Geometry: final body of the model. Coordinates: model frame, mm. Face numbers are marked on the shaded views. Give positions to 0.01 mm unless a question says otherwise; leave off trailing zeros. Write each loop counter-clockwise with the first axis right and the second up, starting at its lowest first coordinate (ties: lowest second). Pieces come first, ordered by that corner, then holes. Notation, with made-up numbers: M 38.25,52 L 49.25,52 A24 cw 49.25,84 Z; hole C 25.25,49 d7. An arc over 180 degrees is marked long. Use a Markdown table: item, result. Add a question column.
1) Section A-A on y = -37. Return the cut outline in (x, z), then the cut area to 3 significant figures.
2) Draft query along X for the marked faces 1, 2, 3 and 4. Return one class per face: +X half, -X half, draft (parallel to the pull), parting line (faces both ways), or undercut.
3) Section D-D on x = 15.5. Return the cut outline in (y, z).
4) Pin query (flat end, axial travel): pin 1 (7 mm diameter, centred on y = -28, z = 61, fed in from -X); pin 2 (1 mm diameter, centred on y = -32.5, z = 47, fed in from +X); pin 3 (12 mm diameter, centred on x = 28, y = -5, fed in from -Z); pin 4 (3 mm diameter, centred on x = 15, y = -7, fed in from -Z). Return the tip coordinate at first contact, or that it passes through.
5) Section C-C on x = -26. Return the cut outline in (y, z), then the cut area to 3 significant figures.
6) Section B-B on z = 59.75. Return the cut outline in (x, y).
7) Line query: line 1 (Y direction, x = 0, z = 55.75); line 2 (X direction, y = -15, z = 50.75); line 3 (X direction, y = -42.5, z = 44). Output: solid intervals per line, ascending.
```python
from build123d import *

# Parameters (mm, degrees)
F3_DEPTH  = 50
F7_DEPTH  = 10
F9_D      = 4.2
F9_DEPTH  = 4.8
F9_TIP    = 1.2618073
F11_D     = 7
F11_DEPTH = 28
F11_TIP   = 2.1030121666


with BuildPart() as f3:
    # F2 (on Front) → F3 (new body)
    with BuildSketch(Plane.XZ):
        with BuildLine():
            ThreePointArc((-26.8236083475, 42.1046311493), (-13.9699038675, 47.9285688805), (0, 49.923))
            Line((0, 49.923), (0, 59))
            Line((0, 59), (-7.5, 59))
            Line((-7.5, 59), (-7.5, 65.5724789832))
            ThreePointArc((-7.5, 65.5724789832), (-22.044813763, 62.2095345277), (-35.4617741509, 55.6638354237))
            Line((-35.4617741509, 55.6638354237), (-26.8236083475, 42.1046311493))
        make_face()
        with BuildLine():
            ThreePointArc((0, 49.923), (13.9699038675, 47.9285688805), (26.8236083475, 42.1046311493))
            Line((26.8236083475, 42.1046311493), (35.4617741509, 55.6638354237))
            ThreePointArc((35.4617741509, 55.6638354237), (22.044813763, 62.2095345277), (7.5, 65.5724789832))
            Line((7.5, 65.5724789832), (7.5, 59))
            Line((7.5, 59), (0, 59))
            Line((0, 59), (0, 49.923))
        make_face()
    extrude(amount=F3_DEPTH)

    # F6 (on line) → F7 (cut)
    with BuildSketch(Plane(origin=(20.9552129656, 0, 45.1351855936), x_dir=(0.9070121064, 0, -0.4211045463), z_dir=(0.4211045463, 0, 0.9070121064))):
        with BuildLine():
            ThreePointArc((3, -47.5), (3.7071067812, -47.2071067812), (4, -46.5))
            Line((4, -46.5), (4, -3.5))
            ThreePointArc((4, -3.5), (3.7071067812, -2.7928932188), (3, -2.5))
            Line((3, -2.5), (-3, -2.5))
            ThreePointArc((-3, -2.5), (-3.7071067812, -2.7928932188), (-4, -3.5))
            Line((-4, -3.5), (-4, -46.5))
            ThreePointArc((-4, -46.5), (-3.7071067812, -47.2071067812), (-3, -47.5))
            Line((-3, -47.5), (3, -47.5))
        make_face()
    extrude(amount=F7_DEPTH, mode=Mode.SUBTRACT)

    # F9
    with Locations(Plane.XY.offset(59)):
        with Locations((0, -25)):
            Hole(F9_D / 2, depth=F9_DEPTH)
            with Locations((0, 0, -(F9_DEPTH + F9_TIP / 2))):  # 118° drill point
                Cone(0, F9_D / 2, F9_TIP, mode=Mode.SUBTRACT)

    # F11
    with Locations(Plane.XZ.offset(50)):
        with Locations((23.4093313461, 50.6118115303)):
            Hole(F11_D / 2, depth=F11_DEPTH)
            with Locations((0, 0, -(F11_DEPTH + F11_TIP / 2))):  # 118° drill point
                Cone(0, F11_D / 2, F11_TIP, mode=Mode.SUBTRACT)


solid = f3.part
```
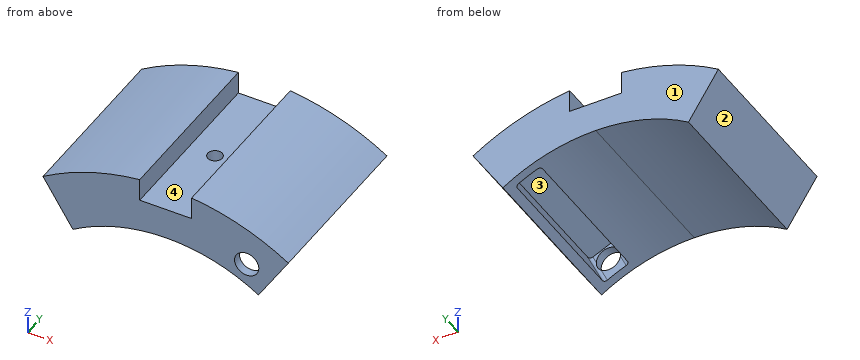
Found:
| question | item | result |
|---|---|---|
| 1 | outline | M -35.46,55.66 L -26.82,42.1 A49.92 cw 17.33,46.82 L 21.54,55.89 L 28.79,52.52 L 24.58,43.45 A49.92 cw 26.82,42.1 L 35.46,55.66 A66 ccw 7.5,65.57 L 7.5,59 L -7.5,59 L -7.5,65.57 A66 ccw Z |
| 1 | area | 875 mm² |
| 2 | face 1 | draft |
| 2 | face 2 | -X half |
| 2 | face 3 | undercut |
| 2 | face 4 | undercut |
| 3 | outline | M -50,47.46 L 0,47.46 L 0,64.15 L -50,64.15 Z |
| 4 | pin 1 | x = -32.4 |
| 4 | pin 2 | x = 30.26 |
| 4 | pin 3 | z = 42.1 |
| 4 | pin 4 | z = 47.12 |
| 5 | outline | M -50,42.62 L 0,42.62 L 0,60.66 L -50,60.66 Z |
| 5 | area | 902 mm² |
| 6 | outline | M -28.03,-50 L -7.5,-50 L -7.5,0 L -28.03,0 Z; M 7.5,-50 L 28.03,-50 L 28.03,0 L 7.5,0 Z |
| 7 | line 1 | -50 to -27.1, -22.9 to 0 |
| 7 | line 2 | -32.33 to 19.15, 27.97 to 32.33 |
| 7 | line 3 | -28.03 to -23.59, 24.84 to 28.03 |
